Design review of the part built by this model. Coordinates are the model's own, in mm. Face numbers are marked on the shaded views. Give positions to 0.01 mm unless a question says otherwise; leave off trailing zeros. Order: outer loops, then holes, each group sorted by start corner. A loop starts at its lowest first (then second) coordinate and runs counter-clockwise, first axis right, second up. Notation, with made-up numbers: M 2,-9.75 L 9,-9.75 A20 cw 9,1.25 Z; hole C 57.5,50.25 d5. An arc over 180 degrees is marked long. Answer as a JSON object with one key per item and string values.
Autodesk Inventor part; units mm, degrees
ref_plane "MUTTER_XY" through (0, 0, 0) normal (0, 0, 1) x (1, 0, 0)
ref_plane "MUTTER_YZ" through (0, 0, 0) normal (1, 0, 0) x (0, 1, 0)
ref_plane "MUTTER_ZX" through (0, 0, 0) normal (0, 1, 0) x (0, 0, 1)
sketch "Sketch_3" plane through (0, 0, 0) normal (1, 0, 0) x (0, 0, -1)
  line L0 (0, 0) -> (-8, 0)
  line L1 (-8, 0) -> (-8, 12)
  line L2 (-8, 12) -> (-7.3569, 14.4)
  line L3 (-7.3569, 14.4) -> (-0.6431, 14.4)
  line L4 (-0.6431, 14.4) -> (0, 12)
  line L5 (0, 12) -> (0, 0)
  line L6 (0, 0) -> (-8, 0)
revolve "Revolution1" add sketch "Sketch_3" angle 360 about axis through (0, 0, 0) along (0, 0, -1)
sketch "Sketch_2" plane through (0, 0, 0) normal (1, 0, 0) x (0, 0, -1)
  line L0 (0, 0) -> (-8, 0)
  line L1 (-8, 0) -> (-8, 8)
  line L2 (-8, 8) -> (-6.9175, 6.9175)
  line L3 (-6.9175, 6.9175) -> (-1.0825, 6.9175)
  line L4 (-1.0825, 6.9175) -> (0, 8)
  line L5 (0, 8) -> (0, 0)
  line L6 (0, 0) -> (-8, 0)
revolve "Revolution2" cut sketch "Sketch_2" angle 360 about axis through (0, 0, 0) along (0, 0, -1)
thread "Thread1"
sketch "Sketch_1" plane through (0, 0, 0) normal (0, 0, 1) x (1, 0, 0)
  line L0 (-24, -24) -> (24, -24)
  line L1 (24, -24) -> (24, 24)
  line L2 (24, 24) -> (-24, 24)
  line L3 (-24, 24) -> (-24, -24)
  line L4 (-12, -6.9282) -> (0, -13.8564)
  line L5 (0, -13.8564) -> (12, -6.9282)
  line L6 (12, -6.9282) -> (12, 6.9282)
  line L7 (12, 6.9282) -> (0, 13.8564)
  line L8 (0, 13.8564) -> (-12, 6.9282)
  line L9 (-12, 6.9282) -> (-12, -6.9282)
extrude "Extrusion1" cut sketch "Sketch_1" along normal blind 8
ref_plane "MUTTER_XY" through (0, 0, 0) normal (0, 0, 1) x (1, 0, 0)
ref_plane "MUTTER_YZ" through (0, 0, 0) normal (1, 0, 0) x (0, 1, 0)
ref_plane "MUTTER_ZX" through (0, 0, 0) normal (0, 1, 0) x (0, 0, 1)
properties part number "SLZ_63_Mutter_M16#"
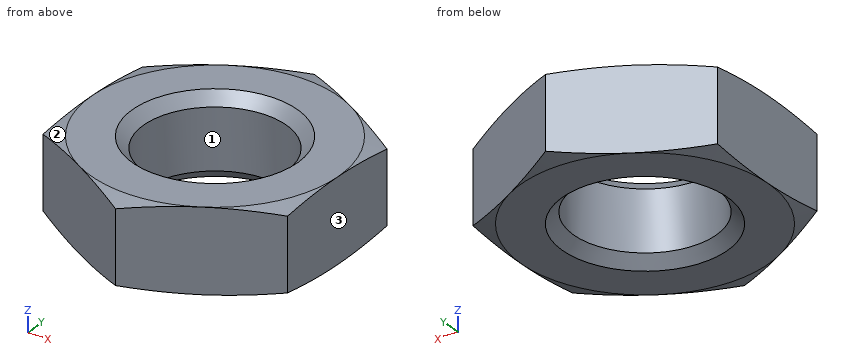
(1) Insertion check: pin 1 (1 mm diameter, centred on x = 8.5, z = 1, fed in from +Y); pin 2 (8.5 mm diameter, centred on x = 0, y = 0, fed in from +Z). Each pin has a flat end and moves straight along its axis. Give the tip position at first contact, or say it passes through.
Checked values:
{"pin 1": "stops at y = 9.24", "pin 2": "passes through"}
(2) To check wall thickness, follow L1, parallel to X at y = 0, z = 6; L2, parallel to Y at x = -2.75, z = 4; L3, parallel to Y at x = -0.5, z = 6.75. State the ranges of each line that lie inside material, in increasing order. Write a range as from..to.
Checked values:
{"L1": "x = -12..-6.92, 6.92..12", "L2": "y = -12.27..-6.35, 6.35..12.27", "L3": "y = -13.57..-6.9, 6.9..13.57"}
(3) We need section A-A (z = 1.5). Write out the cut boundary in (x, y) (1 decimal).
Checked values:
{"outline": "M -12,-6.9 L 0,-13.9 L 12,-6.9 L 12,6.9 L 0,13.9 L -12,6.9 Z; hole C 0,0 d13.8"}
(4) Draft analysis for pull direction X (two halves, no side actions). For the marked faces 1, 2 and 3, state which applies: +X half, -X half, draft (parallel to the pull), parting line (faces both ways), or undercut.
Checked values:
{"face 1": "undercut", "face 2": "-X half", "face 3": "+X half"}
